Autodesk Inventor part; units mm, degrees
ref_plane "YZ Plane" through (0, 0, 0) normal (1, 0, 0) x (0, 1, 0)
ref_plane "XZ Plane" through (0, 0, 0) normal (0, 1, 0) x (-1, 0, 0)
ref_plane "XY Plane" through (0, 0, 0) normal (0, 0, 1) x (1, 0, 0)
sketch "Sketch1" plane through (0, 0, 0) normal (0, 0, 1) x (1, 0, 0)
  line L0 (0, 0) -> (50.8, 0)
  line L1 (-50.8, 101.6) -> (101.6, 101.6)
  line L2 (50.8, 0) -> (78.8, 56)
  line L3 (-28, 56) -> (0, 0)
  line L4 (14.6239, 7) -> (34.6239, 7)
  line L5 (34.6239, 7) -> (34.6239, 2)
  line L6 (34.6239, 2) -> (14.6239, 2)
  line L7 (14.6239, 2) -> (14.6239, 7)
  line L8 (50.8, 0) -> (50.8, 62.4863)
  line L9 (14.6239, 14) -> (34.6239, 14)
  line L10 (34.6239, 14) -> (34.6239, 9)
  line L11 (34.6239, 9) -> (14.6239, 9)
  line L12 (14.6239, 9) -> (14.6239, 14)
  line L13 (14.6239, 21) -> (34.6239, 21)
  line L14 (34.6239, 21) -> (34.6239, 16)
  line L15 (34.6239, 16) -> (14.6239, 16)
  line L16 (14.6239, 16) -> (14.6239, 21)
  line L17 (14.6239, 28) -> (34.6239, 28)
  line L18 (34.6239, 28) -> (34.6239, 23)
  line L19 (34.6239, 23) -> (14.6239, 23)
  line L20 (14.6239, 23) -> (14.6239, 28)
  line L21 (14.6239, 35) -> (34.6239, 35)
  line L22 (34.6239, 35) -> (34.6239, 30)
  line L23 (34.6239, 30) -> (14.6239, 30)
  line L24 (14.6239, 30) -> (14.6239, 35)
  line L25 (14.6239, 42) -> (34.6239, 42)
  line L26 (34.6239, 42) -> (34.6239, 37)
  line L27 (34.6239, 37) -> (14.6239, 37)
  line L28 (14.6239, 37) -> (14.6239, 42)
  circle A0 centre (43.7057, 6.2222) radius 3.1623
  circle A1 centre (43.7057, 28) radius 3.1623
  circle A2 centre (43.7057, 49.7778) radius 3.1623
  line L29 (25.4, 0) -> (25.4, -15.6085)
  circle A3 centre (7.0943, 49.7778) radius 3.1623
  circle A4 centre (7.0943, 6.2222) radius 3.1623
  circle A5 centre (7.0943, 28) radius 3.1623
  line L30 (34.6239, 44) -> (14.6239, 44)
  line L31 (14.6239, 44) -> (14.6239, 49)
  line L32 (34.6239, 49) -> (34.6239, 44)
  line L33 (14.6239, 49) -> (34.6239, 49)
  line L34 (34.6239, 51) -> (14.6239, 51)
  line L35 (14.6239, 51) -> (14.6239, 56)
  line L36 (14.6239, 56) -> (34.6239, 56)
  line L37 (34.6239, 56) -> (34.6239, 51)
  circle A6 centre (-34.29, 91.44) radius 3.1623
  circle A7 centre (85.09, 91.44) radius 3.1623
  line L38 (-28, 56) -> (78.8, 56)
  dimension "d8" = 50.8
  dimension "d9" = 152.4
  dimension "d10" = 101.6
  dimension "d11" = 50.8
  dimension "d12" = 20
  dimension "d13" = 5
  dimension "d14" = 2
  dimension "d15" = 7
  dimension "d16" = 6.3246
  dimension "d17" = 6.3246
  dimension "d18" = 6.3246
  dimension "d19" = 14
  dimension "d20" = 56
  dimension "d21" = 6.2222
  dimension "d22" = 6.2222
  dimension "d23" = 28
  dimension "d24" = 6.3246
  dimension "d25" = 6.3246
  dimension "d26" = 34.29
  dimension "d27" = 34.29
  dimension "d28" = 10.16
  dimension "d29" = 10.16
extrude "Plate1" add sketch "Sketch1" along normal blind 3.048 contours L3 L38 L35 L34 L37 L8 L0 | L8 L38 L2 | L36 L37 L34 L35 | L4 L5 L6 L7 | L9 L10 L11 L12 | L13 L14 L15 L16 | L17 L18 L19 L20 | L21 L22 L23 L24 | L25 L26 L27 L28 | L30 L31 L33 L32
fillet "Corner Round1" radius 6.35 2 edges at (0, 0, 1.524) (50.8, 0, 1.524)
fillet "Corner Round1" radius 3.175 2 edges at (-28, 56, 1.524) (78.8, 56, 1.524)
equation "\"d17\" = d16"
equation "\"d18\" = d17"
equation "\"d21\" = 0.111111 * d20"
equation "\"d22\" = d21"
equation "\"d23\" = 0.5 * d20"
equation "\"d27\" = d26"
equation "\"d29\" = d28"
equation "\"BendRadius\" = Thickness"
equation "\"BendReliefWidth\" = Thickness"
equation "\"BendReliefDepth\" = 0.5 * Thickness"
equation "\"CornerReliefSize\" = 4 * Thickness"
equation "\"MinimumRemnant\" = 2 * Thickness"
equation "\"TransitionRadius\" = BendRadius"
equation "\"JacobiRadiusSize\" = BendRadius"
equation "\"GapSize\" = Thickness"
equation "\"d32\" = BendRadius"
properties part number "Belt plate top"
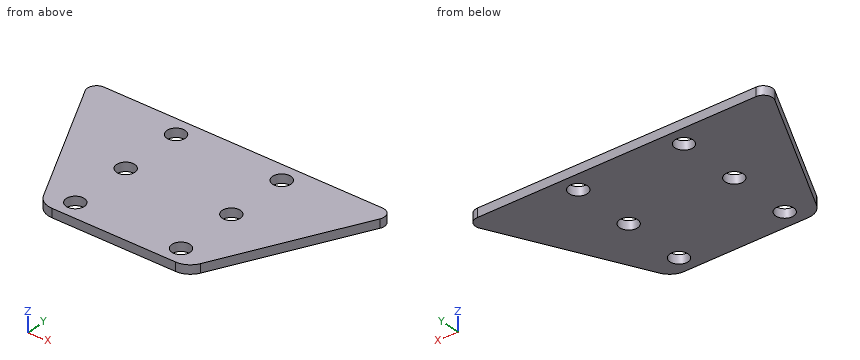
CAD build for the part. Positions are in the model's coordinates, mm. Round coordinates to 2 decimals unless told otherwise and drop trailing zeros. Write each loop counter-clockwise with the first axis right and the second up, starting at its lowest first coordinate (ties: lowest second). Pieces come first, ordered by that corner, then holes. Notation, with made-up numbers: M 88.25,35.25 L 132.25,35.25 A26 cw 132.25,68.25 Z; hole C 59,16 d4. An arc over 180 degrees is marked long. Use a Markdown table: item, result. Add a question column.
1. Slice it at C-C on z = 1.3. Give the cut face in (x, y) (3 decimals), then the cut area to 3 significant figures.
2. Slice it at D-D on x = -6.5. Give the cut face in (y, z).
3. Slice it at B-B on x = 42. Give the cut face in (y, z), then the cut area to 3 significant figures.
4. Flat gauge pin, fed straight in: P1, Ø1, axis at x = 2, z = 0.5, coming from the -Y side. Where does the tip first touch, or does it go through?
5. Drill centre lines: probe 1 along X at (y, z) = (28.5, 0.2); probe 2 along X at (y, z) = (47, 0.9); probe 3 along Y at (x, z) = (-15.5, 2.7). Where is each one in solid material? Low to high.
6. Slice it at A-A on y = 28. Give the cut face in (x, z), then the cut area to 3 significant figures.
Reply:
| question | item | result |
|---|---|---|
| 1 | outline | M -25.703,51.405 L -1.755,3.51 A6.35 ccw 3.925,0 L 46.875,0 A6.35 ccw 52.555,3.51 L 76.503,51.405 A3.175 ccw 73.663,56 L -22.863,56 A3.175 ccw Z; hole C 7.094,6.222 d6.325; hole C 7.094,28 d6.325; hole C 7.094,49.778 d6.325; hole C 43.706,6.222 d6.325; hole C 43.706,28 d6.325; hole C 43.706,49.778 d6.325 |
| 1 | area | 4,210 mm^2 |
| 2 | outline | M 13,0 L 56,0 L 56,3.05 L 13,3.05 Z |
| 3 | outline | M 0,0 L 3.56,0 L 3.56,3.05 L 0,3.05 Z; M 8.89,0 L 25.34,0 L 25.34,3.05 L 8.89,3.05 Z; M 30.66,0 L 47.11,0 L 47.11,3.05 L 30.66,3.05 Z; M 52.44,0 L 56,0 L 56,3.05 L 52.44,3.05 Z |
| 3 | area | 122 mm^2 |
| 4 | P1 | stops at y = 0.16 |
| 5 | probe 1 | x = -14.25 to 3.97, 10.22 to 40.58, 46.83 to 65.05 |
| 5 | probe 2 | x = -23.5 to 5.58, 8.61 to 42.19, 45.22 to 74.3 |
| 5 | probe 3 | y = 31 to 56 |
| 6 | outline | M -14,0 L 3.93,0 L 3.93,3.05 L -14,3.05 Z; M 10.26,0 L 40.54,0 L 40.54,3.05 L 10.26,3.05 Z; M 46.87,0 L 64.8,0 L 64.8,3.05 L 46.87,3.05 Z |
| 6 | area | 202 mm^2 |
